Geometry: final body of the model. Coordinates: model frame, mm. A direction names the side the tool comes from. Round coordinates to 2 decimals unless told otherwise and drop trailing zeros. Loops run counter-clockwise (first coordinate to the right, second up) from the corner with the lowest first, then second, coordinate; pieces in that order, holes last. Notation, with made-up numbers: (-7, -35) - (8, -35) arc R20 cw to (8, 3) - close; hole circle Ø5 at (-10.75, 9.25). An arc over 180 degrees is marked (long way). Write item = value, one per line. Start each with the question number.
Item 1: Section D-D (z = 22.5). Return loops of the section in (x, y), plus the area to 3 significant figures.
Item 2: Draft query along Z for faces 4 (the flat face through (19, 15, 0)), 5 (the flat face through (25.4, 6, 19)), 6 (the flat face through (19, 6, 17.463)). Return one class per face: pulls with the +Z half, pulls with the -Z half, needs draft (parallel to the pull), parting line crosses it, or undercut.
Item 3: Line query: line 1 (Y direction, x = 19.05, z = 1.55); line 2 (Z direction, x = 4.5, y = 13). Output: solid intervals per line, ascending. Write a range as from..to.
Item 4: Access query for faces 1 (the flat face through (19, 7.76, 19)), 2 (the flat face through (19, 0, 21)), 3 (the flat face through (12.7, 6, 19)). Directions: +Z, -Z, +X, -X, +Y, -Y. A direction counts if a zero-diameter tool reaches every point of the face in a straight line with its end or side. Return the directions, or none.
Item 5: Section C-C (x = 7). Return loops of the section in (y, z).
Item 6: First-contact query: pin 1 (8 mm diameter, centred on y = 3, z = 5.5, fed in from -X); pin 2 (2.5 mm diameter, centred on y = 7, z = 19, fed in from +X); pin 3 (2.5 mm diameter, centred on x = 19.05, y = 23.81, fed in from +Z); pin 4 (11.5 mm diameter, centred on x = 19.5, z = 19.5, fed in from +Y). Flat tips, straight axial feed; report the tip coordinate or a pass-through.
Item 7: Section B-B (x = 19.05). Return loops of the section in (y, z), plus the area to 3 significant figures.
Item 8: Section A-A (y = 7). Return loops of the section in (x, z).
from build123d import *

# Parameters (mm, degrees)
BOSS_EXTRUDE1_DEPTH = 38.1
SKETCH2_W           = 12.7
SKETCH2_H           = 3.175
BOSS_EXTRUDE2_DEPTH = 2.9972
SKETCH3_R           = 1.499997
CUT_EXTRUDE1_DEPTH  = 62.749464826


with BuildPart() as part:
    # Sketch1 → Boss-Extrude1 (new body)
    with BuildSketch(Plane(origin=(0, 0, 0), x_dir=(0, 0, -1), z_dir=(1, 0, 0))):
        Polygon((0, 0), (-42.8625, 0), (-42.8625, 4.7625), (-4.7625, 4.7625), (-4.7625, 30.1625), (0, 30.1625), align=None)
    extrude(amount=BOSS_EXTRUDE1_DEPTH)

    # Sketch2 → Boss-Extrude2 (add)
    with BuildSketch(Plane(origin=(0, 4.7625, 0), x_dir=(1, 0, 0), z_dir=(0, 1, 0))):
        with Locations((19.05, -19.05)):
            Rectangle(SKETCH2_W, SKETCH2_H)
    extrude(amount=BOSS_EXTRUDE2_DEPTH)

    # Sketch3 → Cut-Extrude1 (cut, through all)
    with BuildSketch(Plane.XY.offset(4.7625)):
        with Locations((19.05, 23.8125)):
            Circle(SKETCH3_R)
    extrude(amount=-CUT_EXTRUDE1_DEPTH, mode=Mode.SUBTRACT)


solid = part.part
Taken from the geometry:
q1.outline = (0, 0) - (38.1, 0) - (38.1, 4.76) - (0, 4.76) - close
q1.area = 181 mm^2
q2.face_4 = pulls with the -Z half
q2.face_5 = needs draft
q2.face_6 = undercut
q3.line_1 = 0..22.31, 25.31..30.16
q3.line_2 = 0..4.76
q4.face_1 = +Z, +X, -X, +Y
q4.face_2 = +Z, -Z, +X, -X, -Y
q4.face_3 = +Z, -X, +Y
q5.outline = (0, 0) - (30.16, 0) - (30.16, 4.76) - (4.76, 4.76) - (4.76, 42.86) - (0, 42.86) - close
q6.pin_1 = 0
q6.pin_2 = 25.4
q6.pin_3 = through
q6.pin_4 = 7.76
q7.outline = (0, 0) - (22.31, 0) - (22.31, 4.76) - (4.76, 4.76) - (4.76, 17.46) - (7.76, 17.46) - (7.76, 20.64) - (4.76, 20.64) - (4.76, 42.86) - (0, 42.86) - close; (25.31, 0) - (30.16, 0) - (30.16, 4.76) - (25.31, 4.76) - close
q7.area = 320 mm^2
q8.outline = (0, 0) - (38.1, 0) - (38.1, 4.76) - (0, 4.76) - close; (12.7, 17.46) - (25.4, 17.46) - (25.4, 20.64) - (12.7, 20.64) - close
